Could you check a few things on this model? Use its own coordinates, in mm. Face numbers are marked on the shaded views. Round coordinates to 2 decimals unless told otherwise and drop trailing zeros. Loops run counter-clockwise (first coordinate to the right, second up) from the corner with the lowest first, then second, coordinate; pieces in that order, holes last. Notation, with made-up numbers: M -40,68 L 2,68 A17 ccw 2,75 Z; hole C -22,-35.75 d5. An arc over 180 degrees is marked long. Answer in a Markdown table with one row per item.
```python
from build123d import *

# Parameters (mm, degrees)
SALIENTE_EXTRUIR1_DEPTH = 40
CROQUIS2_R              = 10
CORTAR_EXTRUIR1_DEPTH   = 40


with BuildPart() as part:
    # Croquis1 → Saliente-Extruir1 (new body)
    with BuildSketch(Plane.XY):
        Polygon((-18.25, 40), (-13.25, 45), (13.25, 45), (18.25, 40), (18.25, -45), (-18.25, -45), align=None)
    extrude(amount=SALIENTE_EXTRUIR1_DEPTH)

    # Croquis2 → Cortar-Extruir1 (cut)
    with BuildSketch(Plane.XY.offset(40)):
        with Locations((0, 25)):
            Circle(CROQUIS2_R)
        with Locations((0, -15)):
            Circle(CROQUIS2_R)
    extrude(amount=-CORTAR_EXTRUIR1_DEPTH, mode=Mode.SUBTRACT)


solid = part.part
```
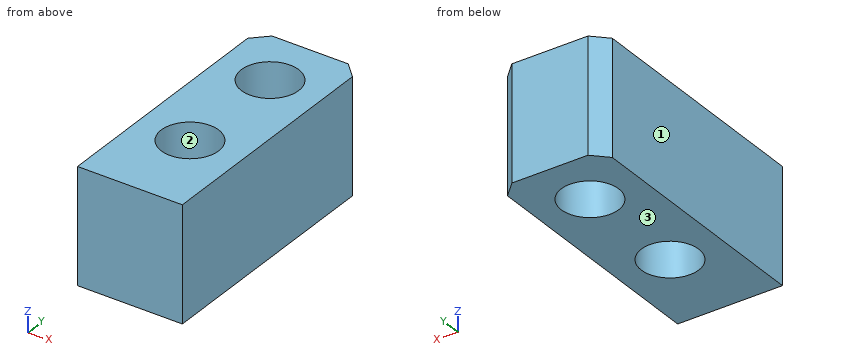
1) I want a section at D-D, the plane y = 18. Please give me the cut outline in (x, z), plus the area to 3 significant figures.
Computed:
| item | result |
|---|---|
| outline | M -18.25,0 L -7.14,0 L -7.14,40 L -18.25,40 Z; M 7.14,0 L 18.25,0 L 18.25,40 L 7.14,40 Z |
| area | 889 mm² |
2) I want a section at B-B, the plane y = -15. Please give me the cut outline in (x, z), plus the area to 3 significant figures.
Computed:
| item | result |
|---|---|
| outline | M -18.25,0 L -10,0 L -10,40 L -18.25,40 Z; M 10,0 L 18.25,0 L 18.25,40 L 10,40 Z |
| area | 660 mm² |
3) If we mould it in two halves opening along X, with no side actions, what happens to the marked faces 1, 2 and 3? For each: released by +X, released by -X, zero draft, split by the parting line, or undercut.
Computed:
| item | result |
|---|---|
| face 1 | released by -X |
| face 2 | undercut |
| face 3 | zero draft |
4) I want a section at C-C, the plane z = 33. Please give me the cut outline in (x, y).
Computed:
| item | result |
|---|---|
| outline | M -18.25,-45 L 18.25,-45 L 18.25,40 L 13.25,45 L -13.25,45 L -18.25,40 Z; hole C 0,-15 d20; hole C 0,25 d20 |
5) I want a section at A-A, the plane x = 0. Please give me the cut outline in (y, z), plus the area to 3 significant figures.
Computed:
| item | result |
|---|---|
| outline | M -45,0 L -25,0 L -25,40 L -45,40 Z; M -5,0 L 15,0 L 15,40 L -5,40 Z; M 35,0 L 45,0 L 45,40 L 35,40 Z |
| area | 2,000 mm² |
6) I need wall thicknesses on line 1 (Y direction, x = 0, z = 16); line 2 (Y direction, x = 1, z = 28.5); line 3 (X direction, y = -19, z = 26). Which ranges of each line are inside material? Lowest first, please.
Computed:
| item | result |
|---|---|
| line 1 | y = -45 to -25, -5 to 15, 35 to 45 |
| line 2 | y = -45 to -24.95, -5.05 to 15.05, 34.95 to 45 |
| line 3 | x = -18.25 to -9.17, 9.17 to 18.25 |
